from build123d import *

# Parameters (mm, degrees)
SKETCH1_W           = 25.4
SKETCH1_H           = 6.35
BOSS_EXTRUDE1_DEPTH = 304.8
SKETCH2_W           = 22.225
SKETCH2_H           = 3.175
CUT_EXTRUDE1_DEPTH  = 306.922412549
CUT_EXTRUDE2_DEPTH  = 306.922412549
CUT_EXTRUDE3_DEPTH  = 306.922412549
SKETCH5_R           = 12.7
BOSS_EXTRUDE2_DEPTH = 6.35
SKETCH6_R           = 9.525
CUT_EXTRUDE4_DEPTH  = 303.759183387


with BuildPart() as part:
    # Sketch1 → Boss-Extrude1 (new body)
    with BuildSketch(Plane.XY):
        with Locations((12.7, 3.175)):
            Rectangle(SKETCH1_W, SKETCH1_H)
    extrude(amount=BOSS_EXTRUDE1_DEPTH)

    # Sketch2 → Cut-Extrude1 (cut, through all)
    with BuildSketch(Plane.XY.offset(304.8)):
        with Locations((12.7, 3.175)):
            Rectangle(SKETCH2_W, SKETCH2_H)
    extrude(amount=-CUT_EXTRUDE1_DEPTH, mode=Mode.SUBTRACT)

    # Sketch3 → Cut-Extrude2 (cut, through all)
    with BuildSketch(Plane.XZ):
        Polygon((20.032348419, 292.1), (16.366174209, 298.45), (9.033825791, 298.45), (5.367651581, 292.1), (9.033825791, 285.75), (16.366174209, 285.75), align=None)
    extrude(amount=-CUT_EXTRUDE2_DEPTH, mode=Mode.SUBTRACT)

    # Sketch4 → Cut-Extrude3 (cut, through all)
    with BuildSketch(Plane(origin=(0, 6.35, 0), x_dir=(1, 0, 0), z_dir=(0, 1, 0))):
        Polygon((0, -288.925), (7.9375, -301.625), (17.4625, -301.625), (25.4, -288.925), (25.4, -304.8), (0, -304.8), align=None)
    extrude(amount=-CUT_EXTRUDE3_DEPTH, mode=Mode.SUBTRACT)

    # Sketch5 → Boss-Extrude2 (add)
    with BuildSketch(Plane(origin=(0, 6.35, 0), x_dir=(1, 0, 0), z_dir=(0, 1, 0))):
        with Locations((12.7, 0)):
            Circle(SKETCH5_R)
    extrude(amount=-BOSS_EXTRUDE2_DEPTH)

    # Sketch6 → Cut-Extrude4 (cut, through all)
    with BuildSketch(Plane(origin=(0, 6.35, 0), x_dir=(1, 0, 0), z_dir=(0, 1, 0))):
        with Locations(Location((12.7, 0, 0), (0, 0, 270))):
            Circle(SKETCH6_R)
    extrude(amount=-CUT_EXTRUDE4_DEPTH, mode=Mode.SUBTRACT)


solid = part.part
Input: part model. Units: mm. Frame: model coordinates. A direction names the side the tool comes from. Give positions to 0.01 mm unless a question says otherwise; leave off trailing zeros. Loops run counter-clockwise (first coordinate to the right, second up) from the corner with the lowest first, then second, coordinate; pieces in that order, holes last. Notation, with made-up numbers: (60, 72.5) -> (70, 72.5) arc R17 cw to (70, 93.5) -> close; hole circle Ø4 at (19.5, -29.5). An arc over 180 degrees is marked (long way). Answer as a JSON object with one key per item and string values. Group by question number.
Item 1: Pin query (flat end, axial travel): P1, Ø1, axis at x = 22.5, y = 3, coming from the +Z side; P2, Ø1.7, axis at x = 11.5, y = 5, coming from the -Z side. Return the tip coordinate at first contact, or that it passes through.
Item 2: Cut plane B-B, the plane x = 12.7. State how many separate pieces and enclosed holes the cut face has, and give its area (3 significant figures).
Item 3: Pull-direction query (Y, two-part tool) for faces 3 (the flat face through (13, 1.588, 156)), 4 (the flat face through (0, 3, 142)), 5 (the flat face through (13, 0, 142)); classes: released by +Y, released by -Y, zero draft, split by the parting line, or undercut.
Item 4: Reachability of faces 1 (the flat face through (13, 4.762, 156)), 2 (the flat face through (13, 6.35, 142)) from +Z, -Z, +X, -X, +Y, -Y: full face, straight path, thin tool, end or side. Return the list, or none.
Item 5: Cut plane A-A, the plane z = 72. Return the cut outline in (x, y), and give its area (3 significant figures).
Item 6: Line query: probe 1 along X at (y, z) = (2.25, 0) (3 decimals); probe 2 along Y at (x, z) = (15.5, 195.5); probe 3 along X at (y, z) = (1.75, 188). Output: solid intervals per line, ascending.
Checks:
{
 "1": {"P1": "stops at z = 8.65", "P2": "stops at z = -12.7"},
 "2": {"separate pieces": "4", "enclosed holes": "0", "area": "917 mm²"},
 "3": {"face 3": "undercut", "face 4": "zero draft", "face 5": "released by -Y"},
 "4": {"face 1": "+Z", "face 2": "+Z, -Z, +X, -X, +Y"},
 "5": {"outline": "(0, 0) -> (25.4, 0) -> (25.4, 6.35) -> (0, 6.35) -> close; hole (1.59, 1.59) -> (23.81, 1.59) -> (23.81, 4.76) -> (1.59, 4.76) -> close", "area": "90.7 mm²"},
 "6": {"probe 1": "x = 0 to 3.175, 22.225 to 25.4", "probe 2": "y = 0 to 1.59, 4.76 to 6.35", "probe 3": "x = 0 to 1.59, 23.81 to 25.4"}
}
